Geometry check sheet. Reference: the model listing, model coordinates, mm. A direction names the side the tool comes from. Round coordinates to 2 decimals unless told otherwise and drop trailing zeros. Order: outer loops, then holes, each group sorted by start corner. A loop starts at its lowest first (then second) coordinate and runs counter-clockwise, first axis right, second up. Notation, with made-up numbers: (77.25, 43.5) - (120.25, 43.5) arc R14 cw to (120.25, 64.5) - close; hole circle Ø2 at (-16.5, -12.5). An arc over 180 degrees is marked (long way). One line per question, with ' | ' between items. Start each with the question number.
Q1. Tool access check on faces 1 (the face through (-125, -19.2, -46.4)), 2 (the face through (2.31, 90.62, -52.45)). Record the directions out of +Z, -Z, +X, -X, +Y, -Y that give a thin tool (end or side, any length) a straight path to the whole face; none if there is none.
Q2. Mould release check, pull along Y, two halves, no side actions. Record for faces 3 (the face through (-1.75, -44.36, -23.07)), 4 (the face through (125, -19.2, -46.4)), 5 (the face through (-19.2, 150, 46.4)), 6 (the face through (1.75, -51.25, 11.38)): +Y half, -Y half, draft (parallel to the pull), parting line (faces both ways), or undercut.
Q3. Sectioned sample at D-D, the plane x = -101. Enter the section's corners in (y, z).
Q4. Gauge pin test, flat ends, axial feed: P1, Ø8, axis at x = 23.5, z = -3.5, coming from the +Y side; P2, Ø4, axis at x = 20.5, y = 73, coming from the +Z side; P3, Ø6, axis at x = 3.5, z = -27.5, coming from the -Y side. Record the tip position at first contact, or that the pin passes through.
Q5. Material ranges on line 1 along X through (y, z) = (132, -2); line 2 along Y through (x, z) = (83.5, 1), recorded low to high.
Q6. Sectioned sample at A-A, the plane z = 0. Enter the section's corners in (x, y).
Q7. Sectioned sample at C-C, the plane y = -21.5. Enter the section's corners in (x, z).
Q8. Sectioned sample at B-B, the plane x = 0. Enter the section's corners in (y, z), then the cut area to 3 significant figures.
```python
from build123d import *
from build123d.topology import SkipClean

# Parameters (mm, degrees)
SKETCH1_R           = 52.5
SKETCH1_R_2         = 50
BOSS_EXTRUDE1_DEPTH = 125
SKETCH2_R           = 52.5
SKETCH2_R_2         = 50
BOSS_EXTRUDE2_DEPTH = 150
CUT_EXTRUDE1_REACH  = 245.696
SKETCH3_R           = 50
SKETCH6_R           = 50
CUT_EXTRUDE2_DEPTH  = 297.236814188


with BuildPart() as part:
    # Sketch1 → Boss-Extrude1 (new, symmetric)
    with BuildSketch(Plane(origin=(0, 0, 0), x_dir=(0, 0, -1), z_dir=(1, 0, 0))):
        Circle(SKETCH1_R)
        Circle(SKETCH1_R_2, mode=Mode.SUBTRACT)
    extrude(amount=BOSS_EXTRUDE1_DEPTH, both=True)

    # Sketch2 → Boss-Extrude2 (add)
    with BuildSketch(Plane(origin=(0, 0, 0), x_dir=(1, 0, 0), z_dir=(0, 1, 0))):
        with Locations(Location((0, 0, 0), (0, 0, 270))):
            Circle(SKETCH2_R)
        with Locations(Location((0, 0, 0), (0, 0, 90))):
            Circle(SKETCH2_R_2, mode=Mode.SUBTRACT)
    extrude(amount=BOSS_EXTRUDE2_DEPTH)

    # Sketch3 → Cut-Extrude1 (cut, up to next)
    with BuildSketch(Plane(origin=(0, 150, 0), x_dir=(1, 0, 0), z_dir=(0, 1, 0)), mode=Mode.PRIVATE) as cut_extrude1_sk1:
        with Locations(Location((0, 0, 0), (0, 0, 270))):
            Circle(SKETCH3_R)
    cut_extrude1_tool1 = extrude(cut_extrude1_sk1.sketch, amount=-CUT_EXTRUDE1_REACH, mode=Mode.PRIVATE) & part.part
    add(cut_extrude1_tool1.solids().sort_by_distance((0, 150, 0))[0], mode=Mode.SUBTRACT)

    # Sketch6 → Cut-Extrude2 (cut, through all)
    with SkipClean():  # the faces are left unmerged after this step: merging them gives an invalid solid
        with BuildSketch(Plane.ZY.offset(125)):
            with Locations(Location((0, 0, 0), (0, 0, 180))):
                Circle(SKETCH6_R)
        extrude(amount=-CUT_EXTRUDE2_DEPTH, mode=Mode.SUBTRACT)


solid = part.part
```
Determined:
1) face 1: +Z, -Z, -X, +Y, -Y | face 2: +Y
2) face 3: undercut | face 4: draft | face 5: +Y half | face 6: parting line
3) outline: circle Ø105 at (0, 0); hole circle Ø100 at (0, 0)
4) P1: stops at y = -49.43 | P2: stops at z = 49.13 | P3: stops at y = -46.43
5) line 1: x = -52.46 to -49.96, 49.96 to 52.46 | line 2: y = -52.49 to -49.99, 49.99 to 52.49
6) outline: (-125, -52.5) - (125, -52.5) - (125, -50) - (-125, -50) - close; (-125, 50) - (-50, 50) - (-50, 150) - (-52.5, 150) - (-52.5, 52.5) - (-125, 52.5) - close; (50, 50) - (125, 50) - (125, 52.5) - (52.5, 52.5) - (52.5, 150) - (50, 150) - close
7) outline: (-125, -47.9) - (125, -47.9) - (125, -45.14) - (-125, -45.14) - close; (-125, 45.14) - (125, 45.14) - (125, 47.9) - (-125, 47.9) - close
8) outline: (0, -52.5) - (150, -52.5) - (150, -50) - (0, -50) arc R50 cw to (0, 50) - (150, 50) - (150, 52.5) - (0, 52.5) arc R52.5 ccw to start | area: 1,150 mm2
